from build123d import *

# Parameters (mm, degrees)
SKETCH1_W                        = 25.3492
SKETCH1_H                        = 7.874
BOSS_EXTRUDE1_DEPTH              = 34.798
CUT_EXTRUDE1_DEPTH               = 8.874
F_97_0_0059_DIAMETER_HOLE1_D     = 5.08
F_97_0_0059_DIAMETER_HOLE1_DEPTH = 12.7
F_97_0_0059_DIAMETER_HOLE1_TIP   = 1.526185972
CHAMFER1_SIZE                    = 0.508
CHAMFER2_SIZE                    = 1.016
DRAFT1_ANGLE                     = -0.25


with BuildPart() as part:
    # Sketch1 → Boss-Extrude1 (new body)
    with BuildSketch(Plane.XY):
        Rectangle(SKETCH1_W, SKETCH1_H)
    extrude(amount=-BOSS_EXTRUDE1_DEPTH)

    # Sketch2 → Cut-Extrude1 (cut, through all)
    with BuildSketch(Plane(origin=(0, 3.937, 0), x_dir=(1, 0, 0), z_dir=(0, 1, 0))):
        Polygon((-2.794, 0), (-2.794, 3.175), (-3.9878, 3.175), (-3.9878, 19.8882), (3.9878, 19.8882), (3.9878, 3.175), (2.794, 3.175), (2.794, 0), align=None)
    extrude(amount=-CUT_EXTRUDE1_DEPTH, mode=Mode.SUBTRACT)

    # #97 (0.0059) Diameter Hole1
    with Locations(Plane.XY):
        with Locations((-8.5852, 0), (8.5852, 0)):
            Hole(F_97_0_0059_DIAMETER_HOLE1_D / 2, depth=F_97_0_0059_DIAMETER_HOLE1_DEPTH)
            with Locations((0, 0, -(F_97_0_0059_DIAMETER_HOLE1_DEPTH + F_97_0_0059_DIAMETER_HOLE1_TIP / 2))):  # 118° drill point
                Cone(0, F_97_0_0059_DIAMETER_HOLE1_D / 2, F_97_0_0059_DIAMETER_HOLE1_TIP, mode=Mode.SUBTRACT)

    # Chamfer1
    chamfer1_edges = [part.edges().sort_by_distance(p)[0] for p in [
        (11.1252, 0, 0),
        (-6.0452, 0, 0),
    ]]
    chamfer(chamfer1_edges, length=CHAMFER1_SIZE)

    # Chamfer2
    chamfer2_edges = [part.edges().sort_by_distance(p)[0] for p in [
        (12.6746, 0, 0),
    ]]
    chamfer(chamfer2_edges, length=CHAMFER2_SIZE)

    # Draft1
    draft1_faces = [part.faces().sort_by_distance(p)[0] for p in [
        (12.1666, 0, -0.508),
        (7.2263, 3.818433137, 0),
        (-5.410856764, 0, 0),
        (0, 0, -34.798),
        (-12.6746, 0, -17.399),
        (12.6746, 0, -17.907),
        (-3.3909, 0, -3.175),
        (3.3909, 0, -3.175),
        (2.794, 0, -1.5875),
        (3.9878, 0, -11.5316),
        (-2.794, 0, -1.5875),
        (0, 0, -19.8882),
        (-3.9878, 0, -11.5316),
    ]]
    draft(draft1_faces, Plane(origin=(-12.6746, 3.937, -34.798), x_dir=(1, 0, 0), z_dir=(0, 1, 0)), DRAFT1_ANGLE)


solid = part.part
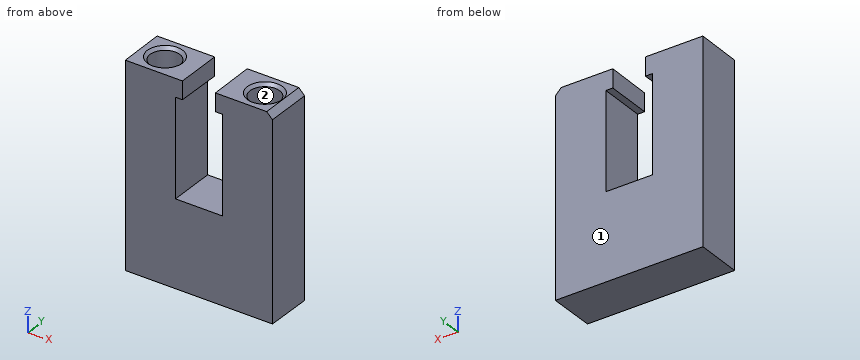
The listing builds one solid part. Answer for the finished solid, in the listing's coordinates (mm). Face numbers are marked on the shaded views. A direction names the side the tool comes from. Give positions to 0.01 mm unless a question says otherwise; leave off trailing zeros. Write each loop counter-clockwise with the first axis right and the second up, starting at its lowest first coordinate (ties: lowest second). Pieces come first, ordered by that corner, then holes.
1) A tool of negligible diameter and unlimited length cuts with its end or side. For the marked faces 1 and 2, from which of +Z, -Z, +X, -X, +Y, -Y can it reach the whole face along a straight path? Write none if from no direction.
2) Find the intervals of material crossed by L1, parallel to X at y = 0, z = -5.5; L2, parallel to X at y = -1.5, z = -7.5; L3, parallel to Z at x = 5.5, y = -1.75, in increasing order.
3) Section B-B (z = -17) is taken. Write down the section's boundary in (x, y), and give its area (3 significant figures).
4) Given P1, Ø3, axis at x = 8.59, y = 0, coming from the -Z side; P2, Ø2, axis at y = 1, z = -29.5, coming from the +X side; P3, Ø2, axis at x = 0, y = 0.5, coming from the +Z side, each flat-ended and moving along its own axis, determine where each tip first touches the part or whether it passes through.
5) Section A-A (z = -6.5) is taken. Write down the section's boundary in (x, y), and give its area (3 significant figures).
Response:
1. face 1: +Z, -Z, +X, -X, +Y
1. face 2: +Z
2. L1: x = -12.66 to -11.13, -6.05 to -4, 4 to 6.05, 11.13 to 12.66
2. L2: x = -12.65 to -10.63, -6.54 to -4.01, 4.01 to 6.54, 10.63 to 12.65
2. L3: z = -34.77 to -0.02
3. outline: (-12.67, 3.94) - (-12.64, -3.94) - (-4.02, -3.94) - (-3.99, 3.94) - close; (3.99, 3.94) - (4.02, -3.94) - (12.64, -3.94) - (12.67, 3.94) - close
3. area: 136 mm2
4. P1: stops at z = -34.79
4. P2: stops at x = 12.67
4. P3: stops at z = -19.9
5. outline: (-12.67, 3.94) - (-12.64, -3.94) - (-4.02, -3.94) - (-3.99, 3.94) - close; (3.99, 3.94) - (4.02, -3.94) - (12.64, -3.94) - (12.67, 3.94) - close; hole circle Ø5.08 at (-8.59, 0); hole circle Ø5.08 at (8.59, 0)
5. area: 95.7 mm2
